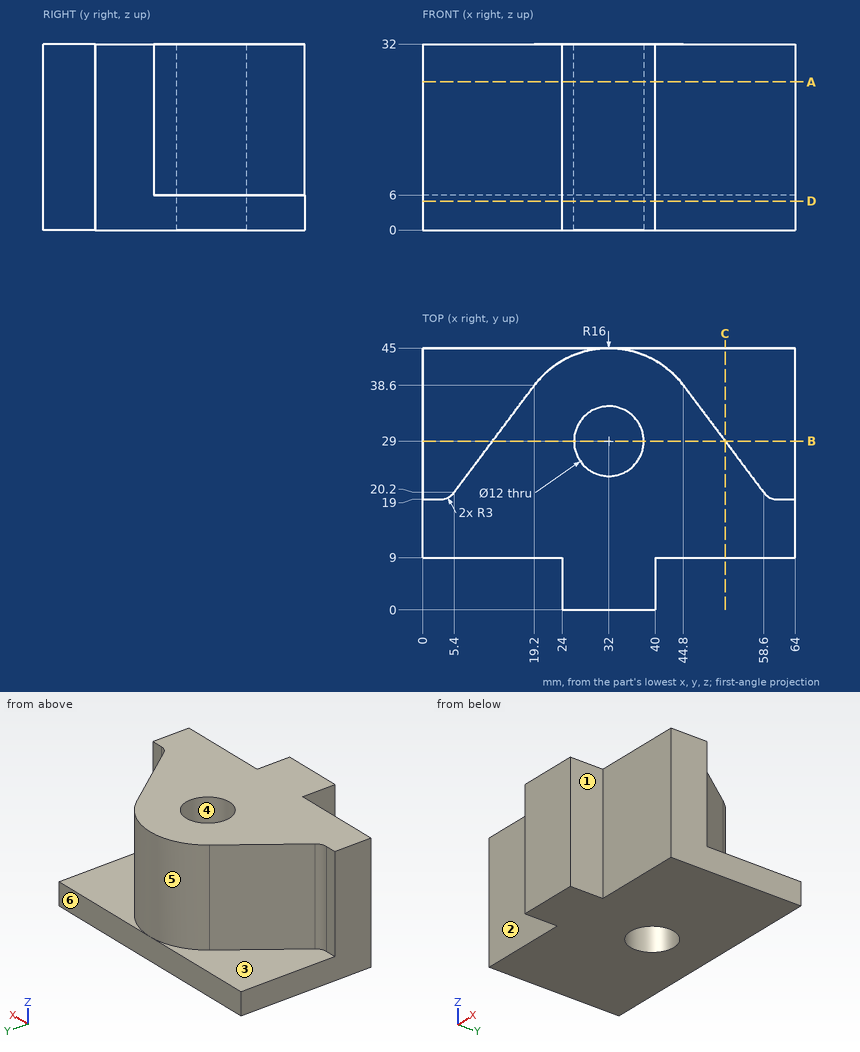
Geometry check sheet. Reference: drawing and pictorial views, mm from the part's lowest x, y, z. A direction names the side the tool comes from. Coordinates: 2 decimals unless noted, no trailing zeros. Write each loop counter-clockwise with the first axis right and the second up, starting at its lowest first coordinate (ties: lowest second). Pieces come first, ordered by that corner, then holes. Notation, with made-up numbers: M 85.5,5 L 121.5,5 A19 cw 121.5,28 Z; hole C 44.25,4 d1. An arc over 180 degrees is marked long. One line per question, with ' | ' between items.
1) Depth check by flat-ended pin: pin 1 Ø7 at (x, y) = (32, 29) entering from -Z; pin 2 Ø3 at (y, z) = (35, 8.5) entering from -X (3 decimals); pin 3 Ø12 at (x, z) = (54.5, 19) entering from -Y; pin 4 Ø1.5 at (x, z) = (1.5, 19) entering from +Y. Enter the tip coordinate at first touch or a pass-through.
Solutions:
pin 1: through | pin 2: x = 15.375 | pin 3: y = 9 | pin 4: y = 19
2) Access from +Z, -Z, +X, -X, +Y, -Y to the whole of each face (thin tool, end or side, straight path). Record for the marked faces 1, 2 and 3.
Solutions:
face 1: +Z, -Z, +X, -Y | face 2: +Z, -Z, -X, -Y | face 3: +Z, -X, +Y
3) Sectioned sample at A-A on z = 25.5. Record the cut outline in (x, y).
Solutions:
outline: M 0,9 L 24,9 L 24,0 L 40,0 L 40,9 L 64,9 L 64,19 L 61,19 A3 cw 58.6,20.2 L 44.8,38.6 A16 ccw 19.2,38.6 L 5.4,20.2 A3 cw 3,19 L 0,19 Z; hole C 32,29 d12
4) Sectioned sample at C-C on x = 52. Record the cut outline in (y, z).
Solutions:
outline: M 9,0 L 45,0 L 45,6 L 29,6 L 29,32 L 9,32 Z
5) Sectioned sample at B-B on y = 29. Record the cut outline in (x, z).
Solutions:
outline: M 0,0 L 26,0 L 26,32 L 12,32 L 12,6 L 0,6 Z; M 38,0 L 64,0 L 64,6 L 52,6 L 52,32 L 38,32 Z
6) Release check for a two-part mould opening along X. For the marked faces 4, 5 and 6 record: +X half, -X half, draft (parallel to the pull), parting line (faces both ways), or undercut.
Solutions:
face 4: undercut | face 5: parting line | face 6: draft
7) Sectioned sample at D-D on z = 5. Record the cut outline in (x, y), then the cut area to 3 significant figures.
Solutions:
outline: M 0,9 L 24,9 L 24,0 L 40,0 L 40,9 L 64,9 L 64,45 L 0,45 Z; hole C 32,29 d12 | area: 2,330 mm^2
8) Material ranges on L1, parallel to Y at x = 32, z = 12.5; L2, parallel to Y at x = 44, z = 3.5; L3, parallel to Y at x = 37, z = 2, recorded low to high.
Solutions:
L1: 0 to 23, 35 to 45 | L2: 9 to 45 | L3: 0 to 25.68, 32.32 to 45
